Geometry: final body of the model. Coordinates: model frame, mm. Face numbers are marked on the shaded views. A direction names the side the tool comes from. Give positions to 0.01 mm unless a question says otherwise; leave off trailing zeros. Write each loop counter-clockwise with the first axis right and the second up, starting at its lowest first coordinate (ties: lowest second). Pieces come first, ordered by that corner, then holes.
from build123d import *

# Parameters (mm, degrees)
BOSS_EXTRU_1_DEPTH      = 20
ESQUISSE1_R             = 1.25
ENL_V_MAT_EXTRU_1_DEPTH = 13.2
ESQUISSE2_W             = 2
ESQUISSE2_H             = 5
ENL_V_MAT_EXTRU_2_DEPTH = 11.5


with BuildPart() as part:
    # ProfileRainureEsquisse → Boss.-Extru.1 (new body)
    with BuildSketch(Plane.XY):
        Polygon((0, 0), (0, 5), (4, 8), (4, 5), (6.2, 5), (6.2, 7.5), (12.2, 7.5), (12.2, -2.5), (6.2, -2.5), (6.2, 0), (4, 0), (4, -3), align=None)
    extrude(amount=BOSS_EXTRU_1_DEPTH)

    # Esquisse1 → Enlèv. mat.-Extru.1 (cut, through all)
    with BuildSketch(Plane(origin=(12.2, 0, 0), x_dir=(0, 0, -1), z_dir=(1, 0, 0))):
        with Locations((-10, 2.5)):
            Circle(ESQUISSE1_R)
    extrude(amount=-ENL_V_MAT_EXTRU_1_DEPTH, mode=Mode.SUBTRACT)

    # Esquisse2 → Enlèv. mat.-Extru.2 (cut, through all)
    with BuildSketch(Plane(origin=(0, 7.5, 0), x_dir=(1, 0, 0), z_dir=(0, 1, 0))):
        with Locations((9.2, -15)):
            Rectangle(ESQUISSE2_W, ESQUISSE2_H)
        with Locations((9.2, -5)):
            Rectangle(ESQUISSE2_W, ESQUISSE2_H)
    extrude(amount=-ENL_V_MAT_EXTRU_2_DEPTH, mode=Mode.SUBTRACT)


solid = part.part
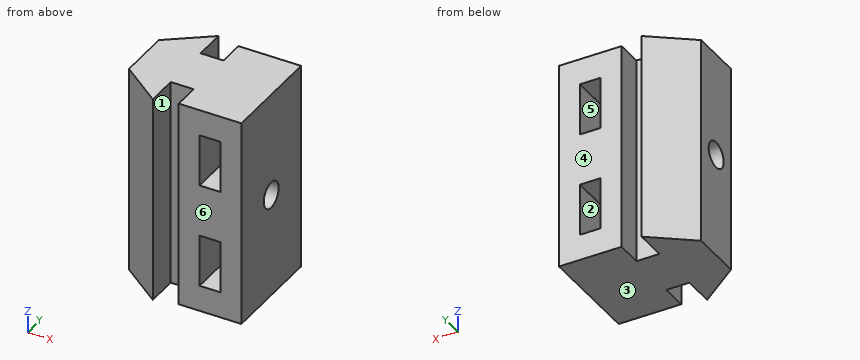
Q1. Section B-B on z = 4. Output: boundary loops of the cut face in (x, y), plus the area to 3 significant figures.
Filled sheet:
outline: (0, 0) - (4, -3) - (4, 0) - (6.2, 0) - (6.2, -2.5) - (8.2, -2.5) - (8.2, 7.5) - (6.2, 7.5) - (6.2, 5) - (4, 5) - (4, 8) - (0, 5) - close; (10.2, -2.5) - (12.2, -2.5) - (12.2, 7.5) - (10.2, 7.5) - close
area: 83.0 mm2
Q2. Section C-C on y = 2.5. Output: boundary loops of the cut face in (x, z).
Filled sheet:
outline: (0, 0) - (12.2, 0) - (12.2, 8.75) - (0, 8.75) - close; (0, 11.25) - (12.2, 11.25) - (12.2, 20) - (0, 20) - close; hole (8.2, 2.5) - (10.2, 2.5) - (10.2, 7.5) - (8.2, 7.5) - close; hole (8.2, 12.5) - (10.2, 12.5) - (10.2, 17.5) - (8.2, 17.5) - close
Q3. Ray query, line 1 along Z through (x, y) = (8.5, 1); line 2 along Y through (x, z) = (8.5, 10); line 3 along Z through (x, y) = (10, 3.25). Return the intervals inside material, ascending.
Filled sheet:
line 1: z = 0 to 2.5, 7.5 to 12.5, 17.5 to 20
line 2: y = -2.5 to 1.25, 3.75 to 7.5
line 3: z = 0 to 2.5, 7.5 to 9, 11 to 12.5, 17.5 to 20
Q4. Section A-A on x = 8.75. Output: boundary loops of the cut face in (y, z), plus the area to 3 significant figures.
Filled sheet:
outline: (-2.5, 0) - (7.5, 0) - (7.5, 2.5) - (-2.5, 2.5) - close; (-2.5, 7.5) - (7.5, 7.5) - (7.5, 12.5) - (-2.5, 12.5) - close; (-2.5, 17.5) - (7.5, 17.5) - (7.5, 20) - (-2.5, 20) - close; hole circle Ø2.5 at (2.5, 10)
area: 95.1 mm2
Q5. Pull-direction query (Z, two-part tool) for the marked faces 1, 2 and 3; classes: released by +Z, released by -Z, zero draft, split by the parting line, or undercut.
Filled sheet:
face 1: zero draft
face 2: undercut
face 3: released by -Z
Q6. Access query for the marked faces 4, 5 and 6. Directions: +Z, -Z, +X, -X, +Y, -Y. A direction counts if a zero-diameter tool reaches every point of the face in a straight line with its end or side. Return the directions, or none.
Filled sheet:
face 4: +Z, -Z, +X, +Y
face 5: +Y, -Y
face 6: +Z, -Z, +X, -Y
Q7. Section D-D on x = 11.25. Output: boundary loops of the cut face in (y, z).
Filled sheet:
outline: (-2.5, 0) - (7.5, 0) - (7.5, 20) - (-2.5, 20) - close; hole circle Ø2.5 at (2.5, 10)
Q8. Pin query (flat end, axial travel): P1, Ø2.5, axis at x = 5.5, z = 13, coming from the +Y side; P2, Ø1.8, axis at x = 5.5, z = 8, coming from the -Y side; P3, Ø0.8, axis at y = -1.5, z = 8, coming from the -X side. Return the tip coordinate at first contact, or that it passes through.
Filled sheet:
P1: stops at y = 7.5
P2: stops at y = -2.5
P3: stops at x = 1.47
